Answer from the drawing. Dimensions are ordinates in mm from the lowest x, y and z of the part. Give positions to 0.01 mm unless a question says otherwise; leave off trailing zeros. Loops run counter-clockwise (first coordinate to the right, second up) from the corner with the lowest first, then second, coordinate; pieces in that order, holes last. Notation, with made-up numbers: (30.5, 4) - (80.5, 4) arc R24 cw to (80.5, 16) - close; hole circle Ø9 at (58, 31). An arc over 180 degrees is marked (long way). Put each result on its own line as item: value. Start each with the question number.
1. Given pin 1 Ø4 at (y, z) = (23.5, 4) entering from +X; pin 2 Ø1.5 at (y, z) = (23.5, 3) entering from +X, each flat-ended and moving along its own axis, determine where each tip first touches the part or whether it passes through.
2. A cutting plane is placed at D-D, the plane x = 65. Determine the outline of the cut face in (y, z).
3. For a pull along X with two mould halves and no side action, classify the marked faces 1, 2 and 3 as released by +X, released by -X, zero draft, split by the parting line, or undercut.
4. Consider L1, parallel to X at y = 11.25, z = 4 (1 decimal); L2, parallel to X at y = 20.5, z = 2.25 (1 decimal); L3, parallel to Y at x = 46, z = 0.5. Determine where each line is inside the solid, lowest interval first. Write a range as from..to.
5. A cutting plane is placed at B-B, the plane x = 6.5. Determine the outline of the cut face in (y, z) (1 decimal), plus the area to 3 significant figures.
6. A cutting plane is placed at A-A, the plane z = 5.75. Count the separate pieces of the cut face and the enclosed holes in it, plus the area to 3 significant figures.
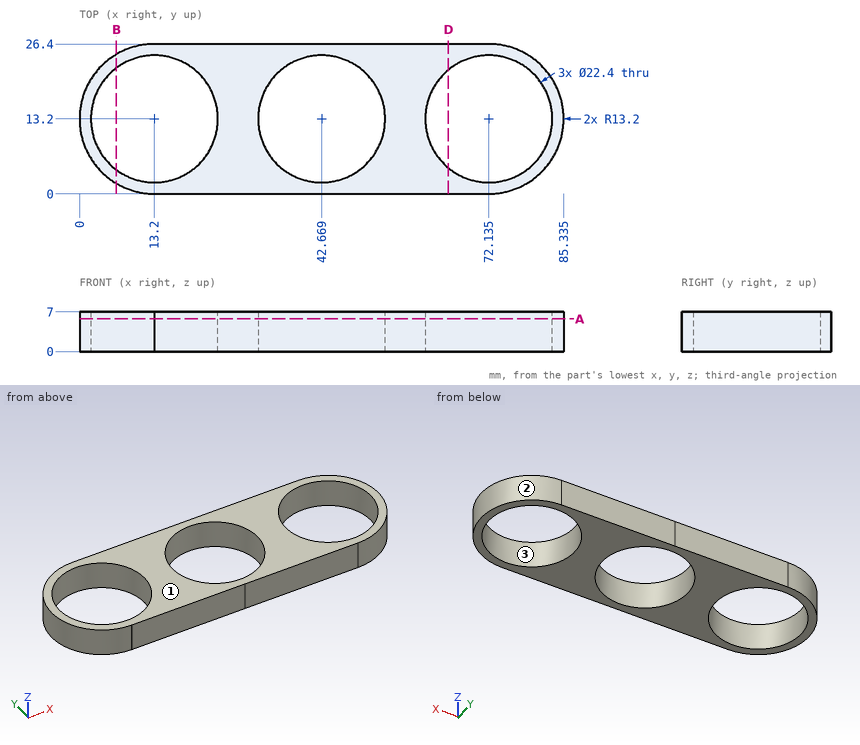
Return value:
1. pin 1: stops at x = 82.4
1. pin 2: stops at x = 81.25
2. outline: (0, 0) - (4.57, 0) - (4.57, 7) - (0, 7) - close; (21.83, 0) - (26.4, 0) - (26.4, 7) - (21.83, 7) - close
3. face 1: zero draft
3. face 2: released by +X
3. face 3: undercut
4. L1: x = 0.1..2.2, 24.2..31.6, 53.7..61.1, 83.2..85.2
4. L2: x = 2.2..4.7, 21.7..34.2, 51.2..63.6, 80.6..83.1
4. L3: y = 0..2.51, 23.89..26.4
5. outline: (1.8, 0) - (4.2, 0) - (4.2, 7) - (1.8, 7) - close; (22.2, 0) - (24.6, 0) - (24.6, 7) - (22.2, 7) - close
5. area: 33.6 mm2
6. separate pieces: 1
6. enclosed holes: 3
6. area: 921 mm2
